from build123d import *

# Parameters (mm, degrees)
SKETCH1_W           = 295
SKETCH1_H           = 295
BOSS_EXTRUDE1_DEPTH = 6.35
SKETCH2_W           = 100
SKETCH2_H           = 100
BOSS_EXTRUDE2_DEPTH = 10
SKETCH6_W           = 10
SKETCH6_H           = 100
CUT_EXTRUDE1_DEPTH  = 5


# Read off the part's stored shape, not the designer's step: CSK for M6 Flat Head Machine Screw1
with BuildPart() as part:
    # Sketch1 → Boss-Extrude1 (new body)
    with BuildSketch(Plane.XY):
        with Locations((147.5, 147.5)):
            Rectangle(SKETCH1_W, SKETCH1_H)
    extrude(amount=BOSS_EXTRUDE1_DEPTH)

    # Sketch2 → Boss-Extrude2 (add)
    with BuildSketch(Plane.XY.offset(6.35)):
        with Locations((295, 147.5)):
            Rectangle(SKETCH2_W, SKETCH2_H)
    extrude(amount=BOSS_EXTRUDE2_DEPTH)

    # CSK for M6 Flat Head Machine Screw1 outl → CSK for M6 Flat Head Machine Screw1 (revolve, cut)
    with BuildSketch(Plane(origin=(325, 177.5, 0), x_dir=(1, 0, 0), z_dir=(0, -1, 0))):
        Polygon((0, 6.35), (3.2, 6.35), (3.2, 13.25), (6.3, 16.35), (0, 16.35), align=None)
    revolve(axis=Axis((325, 177.5, 0), (0, 0, 1)), mode=Mode.SUBTRACT)

    # CSK for M6 Flat Head Machine Screw1 2 ou → CSK for M6 Flat Head Machine Screw1 2 (revolve, cut)
    with BuildSketch(Plane(origin=(265, 117.5, 0), x_dir=(1, 0, 0), z_dir=(0, -1, 0))):
        Polygon((0, 16.35), (0, 4.427246019), (3.2, 6.35), (3.2, 13.25), (6.3, 16.35), align=None)
    revolve(axis=Axis((265, 117.5, 0), (0, 0, 1)), mode=Mode.SUBTRACT)

    # CSK for M6 Flat Head Machine Screw1 3 ou → CSK for M6 Flat Head Machine Screw1 3 (revolve, cut)
    with BuildSketch(Plane(origin=(325, 117.5, 0), x_dir=(1, 0, 0), z_dir=(0, -1, 0))):
        Polygon((0, 6.35), (3.2, 6.35), (3.2, 13.25), (6.3, 16.35), (0, 16.35), align=None)
    revolve(axis=Axis((325, 117.5, 0), (0, 0, 1)), mode=Mode.SUBTRACT)

    # CSK for M6 Flat Head Machine Screw1 4 ou → CSK for M6 Flat Head Machine Screw1 4 (revolve, cut)
    with BuildSketch(Plane(origin=(265, 177.5, 0), x_dir=(1, 0, 0), z_dir=(0, -1, 0))):
        Polygon((0, 16.35), (0, 4.427246019), (3.2, 6.35), (3.2, 13.25), (6.3, 16.35), align=None)
    revolve(axis=Axis((265, 177.5, 0), (0, 0, 1)), mode=Mode.SUBTRACT)

    # Sketch6 → Cut-Extrude1 (cut)
    with BuildSketch(Plane.XY.offset(16.35)):
        with Locations((295, 147.5)):
            Rectangle(SKETCH6_W, SKETCH6_H)
    extrude(amount=-CUT_EXTRUDE1_DEPTH, mode=Mode.SUBTRACT)


solid = part.part
Work out the finished part from the listing and answer in its coordinate system (mm). A direction names the side the tool comes from. Round coordinates to 2 decimals unless told otherwise and drop trailing zeros. Loops run counter-clockwise (first coordinate to the right, second up) from the corner with the lowest first, then second, coordinate; pieces in that order, holes last. Notation, with made-up numbers: M 74.25,-24.5 L 91.25,-24.5 A21 cw 91.25,-11.5 Z; hole C 51.5,32 d1. An arc over 180 degrees is marked long. One line per question, with ' | ' between items. Start each with the question number.
(1) A cutting plane is placed at B-B on x = 226. Write down the section's boundary in (y, z), plus the area to 3 significant figures.
(2) Flat-ended cylindrical pins translate along their axes: pin 1 Ø2 at (x, y) = (216, 202) entering from +Z; pin 2 Ø5 at (x, z) = (310.5, 9) entering from +Y; pin 3 Ø6 at (x, z) = (215, 7.5) entering from -Y; pin 4 Ø3 at (x, y) = (295.5, 143.5) entering from +Z. Find the tip coordinate at first contact, or state that the pin passes through.
(3) A tool of negligible diameter and unlimited length cuts with its end or side. For faces 5 (the face through (294, 97.5, 11)), 6 (the face through (245, 147, 11)), 7 (the face through (267, 148, 16.35)), 8 (the face through (320, 148, 6.35)), 9 (the face through (264.26, 174.19, 13.44)), from which of +Z, -Z, +X, -X, +Y, -Y can it reach the whole face along a straight path? Write none if from no direction.
(4) For a pull along Y with two mould halves and no side action, classify faces 1 (the face through (294, 197.5, 11)), 2 (the face through (321.609, 177.649, 13.444)), 3 (the face through (295, 148, 11.35)), 4 (the face through (266.566, 114.489, 13.444)) as released by +Y, released by -Y, zero draft, split by the parting line, or undercut.
(5) Find the intervals of material crossed by line 1 (X direction, y = 177.5, z = 8.25); line 2 (Y direction, x = 265, z = 8.5); line 3 (X direction, y = 117.5, z = 13.75), in increasing order.
(6) A cutting plane is placed at A-A on y = 152. Write down the section's boundary in (x, z).
Geometry check:
1) outline: M 0,0 L 295,0 L 295,6.35 L 0,6.35 Z | area: 1,870 mm²
2) pin 1: stops at z = 6.35 | pin 2: stops at y = 197.5 | pin 3: stops at y = 0 | pin 4: stops at z = 11.35
3) face 5: +Z, +X, -X, -Y | face 6: +Z, -X, +Y, -Y | face 7: +Z, +X, -X, +Y, -Y | face 8: -Z, +X, +Y, -Y | face 9: +Z
4) face 1: released by +Y | face 2: undercut | face 3: zero draft | face 4: undercut
5) line 1: x = 245 to 261.8, 268.2 to 321.8, 328.2 to 345 | line 2: y = 97.5 to 114.3, 120.7 to 174.3, 180.7 to 197.5 | line 3: x = 245 to 261.3, 268.7 to 290, 300 to 321.3, 328.7 to 345
6) outline: M 0,0 L 295,0 L 295,6.35 L 345,6.35 L 345,16.35 L 300,16.35 L 300,11.35 L 290,11.35 L 290,16.35 L 245,16.35 L 245,6.35 L 0,6.35 Z
